Geometry check sheet. Reference: the model listing, model coordinates, mm. Face numbers are marked on the shaded views. A direction names the side the tool comes from. Round coordinates to 2 decimals unless told otherwise and drop trailing zeros. Order: outer loops, then holes, each group sorted by start corner. A loop starts at its lowest first (then second) coordinate and runs counter-clockwise, first axis right, second up. Notation, with made-up numbers: (-14, 39) - (42, 39) arc R10 ccw to (42, 46) - close; hole circle Ø10 at (77.5, -32). An arc over 180 degrees is marked (long way). Write each question's results on one line, items separated by ' | '.
```python
from build123d import *

# Parameters (mm, degrees)
SKETCH10_R          = 2.5
BOSS_EXTRUDE3_DEPTH = 10
SKETCH10_3_R        = 15
SKETCH10_3_R_2      = 10
BOSS_EXTRUDE4_DEPTH = 30
FILLET1_RADIUS      = 25
FILLET1_LENGTH      = 10
FILLET2_R           = 20
CUT_EXTRUDE1_START  = 25
SKETCH10_6_R        = 15
SKETCH10_6_R_2      = 10
CUT_EXTRUDE1_DEPTH  = 5


with BuildPart() as part:
    # Sketch10 → Boss-Extrude3 (new body)
    with BuildSketch(Plane(origin=(0, 0, 0), x_dir=(1, 0, 0), z_dir=(0, 1, 0))):
        with BuildLine():
            ThreePointArc((44.364916731, 20), (5, 25), (44.364916731, 30))
            Line((44.364916731, 30), (95, 30))
            Line((95, 30), (95, 50))
            Line((95, 50), (0, 50))
            Line((0, 50), (0, 0))
            Line((0, 0), (95, 0))
            Line((95, 0), (95, 20))
            Line((95, 20), (44.364916731, 20))
        make_face()
        with Locations(Location((80, 15, 0), (0, 0, 270))):
            Circle(SKETCH10_R, mode=Mode.SUBTRACT)
        with Locations(Location((80, 35, 0), (0, 0, 270))):
            Circle(SKETCH10_R, mode=Mode.SUBTRACT)
    extrude(amount=BOSS_EXTRUDE3_DEPTH)

    # Sketch10<3> → Boss-Extrude4 (add)
    # profile 1 of 2: a face of its own
    with BuildSketch(Plane(origin=(0, 0, 0), x_dir=(1, 0, 0), z_dir=(0, 1, 0))):
        with BuildLine():
            Line((95, 30), (44.364916731, 30))
            ThreePointArc((44.364916731, 30), (5, 25), (44.364916731, 20))
            Line((44.364916731, 20), (95, 20))
            Line((95, 20), (95, 30))
        make_face()
        with Locations((25, 25)):
            Circle(SKETCH10_3_R, mode=Mode.SUBTRACT)
    # profile 2 of 2: a face of its own
    with BuildSketch(Plane(origin=(0, 0, 0), x_dir=(1, 0, 0), z_dir=(0, 1, 0))):
        with Locations((25, 25)):
            Circle(SKETCH10_3_R)
        with Locations(Location((25, 25, 0), (0, 0, 270))):
            Circle(SKETCH10_3_R_2, mode=Mode.SUBTRACT)
    extrude(amount=BOSS_EXTRUDE4_DEPTH)

    # Fillet1: full round fillet: the end face becomes a half cylinder, R = half its width
    fillet1_face = Plane((0, 5, -25), x_dir=(0, 1, 0), z_dir=(-1, 0, 0))  # on the end face: x along it, z out of the body
    fillet1_slab = fillet1_face.offset(-FILLET1_RADIUS / 2) * Box(FILLET1_LENGTH, 2 * FILLET1_RADIUS, FILLET1_RADIUS, mode=Mode.PRIVATE)  # the body's end, R deep
    fillet1_round = Plane((25, 5, -25), x_dir=(-1, 0, 0), z_dir=(0, 1, 0)) * Cylinder(FILLET1_RADIUS, FILLET1_LENGTH, mode=Mode.PRIVATE)  # its axis R under the face
    add(fillet1_slab - fillet1_round, mode=Mode.SUBTRACT)

    # Fillet2
    fillet2_edges = [part.edges().sort_by_distance(p)[0] for p in [
        (95, 30, -25),
    ]]
    fillet(fillet2_edges, radius=FILLET2_R)

    # Sketch10<6> → Cut-Extrude1 (cut)
    with BuildSketch(Plane(origin=(0, 0, 0), x_dir=(1, 0, 0), z_dir=(0, 1, 0)).offset(CUT_EXTRUDE1_START)):
        with Locations(Location((25, 25, 0), (0, 0, 270))):
            Circle(SKETCH10_6_R)
        with Locations(Location((25, 25, 0), (0, 0, 270))):
            Circle(SKETCH10_6_R_2, mode=Mode.SUBTRACT)
    extrude(amount=CUT_EXTRUDE1_DEPTH, mode=Mode.SUBTRACT)


solid = part.part
```
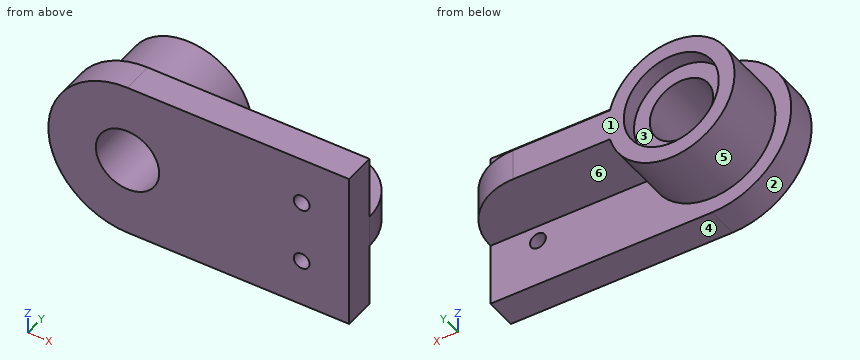
(1) Section check A-A (z = -25). Record the cut outline in (x, y).
Answers follow:
outline: (0, 0) - (15, 0) - (15, 25) - (10, 25) - (10, 30) - (5, 30) - (5, 10) - (0, 10) - close; (35, 0) - (95, 0) - (95, 10) arc R20 ccw to (75, 30) - (40, 30) - (40, 25) - (35, 25) - close
(2) Depth check by flat-ended pin: pin 1 Ø24 at (x, z) = (29, -24.5) entering from +Y; pin 2 Ø10 at (y, z) = (26.5, -14.5) entering from -X; pin 3 Ø10 at (y, z) = (17, -8) entering from +X; pin 4 Ø16 at (x, z) = (25, -25) entering from +Y. Enter the tip coordinate at first touch or a pass-through.
Answers follow:
pin 1: y = 30 | pin 2: x = 5.77 | pin 3: x = 41 | pin 4: through
(3) Section check C-C (y = 7.5). Record the cut outline in (x, z).
Answers follow:
outline: (25, -50) - (95, -50) - (95, 0) - (25, 0) arc R25 ccw to start; hole circle Ø20 at (25, -25); hole circle Ø5 at (80, -35); hole circle Ø5 at (80, -15)
(4) Access from +Z, -Z, +X, -X, +Y, -Y to the whole of each face (thin tool, end or side, straight path). Record for the marked faces 4, 5 and 6.
Answers follow:
face 4: -Z, +X, -X, +Y, -Y | face 5: +Y | face 6: -Z, +X, +Y
(5) Draft check along X on the marked faces 1, 2 and 3. Enter one of: released by +X, released by -X, zero draft, split by the parting line, or undercut.
Answers follow:
face 1: zero draft | face 2: released by -X | face 3: undercut
(6) Section check B-B (x = 26.5). Record the cut outline in (y, z), then the cut area to 3 significant figures.
Answers follow:
outline: (0, -50) - (10, -50) - (10, -44.94) - (30, -44.94) - (30, -39.92) - (25, -39.92) - (25, -34.89) - (0, -34.89) - close; (0, -15.11) - (25, -15.11) - (25, -10.08) - (30, -10.08) - (30, -5.06) - (10, -5.06) - (10, 0) - (0, 0) - close | area: 654 mm²
(7) Material ranges on line 1 (Y direction, x = 56, z = -44.5); line 2 (Z direction, x = 77, y = 22); line 3 (X direction, y = 18, z = -27), recorded low to high.
Answers follow:
line 1: 0 to 10 | line 2: -30 to -20 | line 3: 5.1 to 15.2, 34.8 to 93.33
(8) Section check D-D (x = 47.5). Record the cut outline in (y, z), then the cut area to 3 significant figures.
Answers follow:
outline: (0, -50) - (10, -50) - (10, -30) - (30, -30) - (30, -20) - (10, -20) - (10, 0) - (0, 0) - close | area: 700 mm²
